Geometry check sheet. Reference: the model listing, model coordinates, mm. A direction names the side the tool comes from. Round coordinates to 2 decimals unless told otherwise and drop trailing zeros. Write each loop counter-clockwise with the first axis right and the second up, starting at its lowest first coordinate (ties: lowest second). Pieces come first, ordered by that corner, then holes. Notation, with made-up numbers: M 39.5,24 L 55.5,24 A24 ccw 55.5,44 Z; hole C 62,13.25 d3. An arc over 180 degrees is marked long. Put each result on its own line as item: value. Start each with the question number.
(1) Tool access check on faces 4 (the flat face through (-17.76, -1.35, 2.47)), 5 (the flat face through (-23.755, -34.483, 2.465)), 6 (the cylindrical face through (48.09, 32.49, 6.5)). Record the directions out of +Z, -Z, +X, -X, +Y, -Y that give a thin tool (end or side, any length) a straight path to the whole face; none if there is none.
(2) Mould release check, pull along Y, two halves, no side actions. Record for faces 1 (the cylindrical face through (31.496, 18.9, 6.496)), 2 (the flat face through (94.077, -15.476, 1.521)), 3 (the flat face through (-33.36, 17.06, 3.94)): pulls with the +Y half, pulls with the -Y half, needs draft (parallel to the pull), parting line crosses it, or undercut.
(3) Section check D-D on x = 32. Record the cut outline in (y, z).
(4) Gauge pin test, flat ends, axial feed: pin 1 (1 mm diameter, centred on x = -35, z = 3, fed in from -Y); pin 2 (1.5 mm diameter, centred on x = 19, z = 1, fed in from -Y); pin 3 (3.5 mm diameter, centred on y = 31, z = 2, fed in from -X). Record the tip position at first contact, or that the pin passes through.
(5) Section check A-A on x = -30.5. Record the cut outline in (y, z), then the cut area to 3 significant figures.
(6) Section check C-C on y = -47. Record the cut outline in (x, z).
(7) Section check B-B on z = 1.5. Record the cut outline in (x, y), then the cut area to 3 significant figures.
(8) Material ranges on probe 1 along X at (y, z) = (40.5, 1.25); probe 2 along Y at (x, z) = (-27, 6.5); probe 3 along X at (y, z) = (37, 5.5), recorded low to high.
from build123d import *

# Parameters (mm, degrees)
PAD_DEPTH    = 8
FILLET_R     = 5
CHAMFER_SIZE = 3


with BuildPart() as part:
    # Sketch → Pad (new body)
    with BuildSketch(Plane.XY):
        Polygon((-46.734573, 12.37682), (-22.466158, 20.873907), (-12.919914, -24.196195), (-34.898476, -45.061794), (22.378998, -60.602196), (95.640884, -16.201052), (82.764542, 47.958603), (46.662025, 50.132896), (46.662025, 20.325462), (11.88671, 20.325462), (8.24356, 53.776024), (-50.377705, 53.776024), align=None)
    extrude(amount=PAD_DEPTH)

    # Fillet
    fillet_edges = [part.edges().sort_by_distance(p)[0] for p in [
        (29.274368, 20.325462, 8),
        (46.662025, 35.229179, 8),
        (64.713284, 49.045749, 8),
        (89.202713, 15.878775, 8),
    ]]
    fillet(fillet_edges, radius=FILLET_R)

    # Chamfer
    chamfer_edges = [part.edges().sort_by_distance(p)[0] for p in [
        (56.736601, -39.779406, 8),
        (-6.259739, -52.831995, 8),
        (-23.909195, -34.628995, 8),
        (-17.693036, -1.661144, 8),
    ]]
    chamfer(chamfer_edges, length=CHAMFER_SIZE)


solid = part.part
Answers follow:
1. face 4: +Z, -Z
1. face 5: +Z, -Z, -X
1. face 6: +Z, +Y
2. face 1: pulls with the +Y half
2. face 2: pulls with the -Y half
2. face 3: undercut
3. outline: M -54.77,0 L 20.33,0 L 20.33,3 A5 ccw 15.33,8 L -51.26,8 L -54.77,5 Z
4. pin 1: stops at y = -45.17
4. pin 2: stops at y = -59.89
4. pin 3: stops at x = -48.53
5. outline: M -46.26,0 L -40.89,0 L -40.89,5 L -43.95,7.22 L -46.26,5 Z; M 18.06,0 L 53.78,0 L 53.78,8 L 18.06,8 Z
5. area: 319 mm^2
6. outline: M -27.75,0 L 44.82,0 L 44.82,5 L 39.03,8 L -16.3,8 L -27.75,5 Z
7. outline: M -50.38,53.78 L -46.73,12.38 L -22.47,20.87 L -12.92,-24.2 L -34.9,-45.06 L 22.38,-60.6 L 93.08,-17.76 L 95.05,-13.26 L 82.76,47.96 L 46.66,50.13 L 46.66,20.33 L 11.89,20.33 L 8.24,53.78 Z
7. area: 10,500 mm^2
8. probe 1: x = -49.21 to 9.69, 46.66 to 84.26
8. probe 2: y = -45.65 to -39.63, 19.29 to 53.78
8. probe 3: x = -48.9 to 10.07, 47.33 to 84.28
